Design review of the part built by this model. Coordinates are the model's own, in mm. Coordinates: 2 decimals unless noted, no trailing zeros. Write each loop counter-clockwise with the first axis right and the second up, starting at its lowest first coordinate (ties: lowest second). Pieces come first, ordered by that corner, then holes.
Q1. Add section A-A, the plane x = -35. Give the boundary of the cut face in (y, z), plus the area to 3 significant figures.
Q2. Add section C-C, the plane x = 365. Give the number of separate pieces and of enclosed holes in the cut face, plus the area to 3 significant figures.
Q3. To check wall thickness, follow probe 1 along X at (y, z) = (-37, 244); probe 2 along Z at (x, y) = (-161.5, -37); probe 3 along X at (y, z) = (-2, -305.5). State the ranges of each line that lie inside material, in increasing order.
Q4. Add section B-B, the plane z = -432. Give the boundary of the cut face in (x, y), plus the area to 3 significant figures.
from build123d import *

# Parameters (mm, degrees)
F0_W     = 1080
F0_H     = 2590
F0_W_2   = 20
F0_H_2   = 300
F0_W_3   = 340
F0_H_3   = 40
F0_H_4   = 420
F1_DEPTH = 40


# Not quite as in the source:
# - a feature names something its author has since deleted; it is built from what else it names


with BuildPart() as f1:
    # F0 (on Front) → F1 (new body)
    with BuildSketch(Plane.XZ):
        Rectangle(F0_W, F0_H)
        Polygon((520, -855), (520, -1275), (10, -1275), (-10, -1275), (-520, -1275), (-520, -855), (-520, -795), (-520, -495), (-520, -455), (-520, -155), (-520, -115), (-520, 595), (-520, 635), (-520, 935), (-520, 975), (-520, 1275), (160, 1275), (180, 1275), (520, 1275), (520, 975), (520, 935), (520, 635), (520, 595), (520, 339.328327179), (520, 299.328327179), (520, -115), (520, -155), (520, -455), (520, -495), (520, -795), align=None, mode=Mode.SUBTRACT)
        with Locations((170, 1125)):
            Rectangle(F0_W_2, F0_H_2)
        Polygon((-160, 935), (520, 935), (520, 975), (180, 975), (160, 975), (-520, 975), (-520, 935), (-180, 935), align=None)
        with Locations((-170, 785)):
            Rectangle(F0_W_2, F0_H_2)
        Polygon((180, 595), (520, 595), (520, 635), (-160, 635), (-180, 635), (-520, 635), (-520, 595), (160, 595), align=None)
        Polygon((160, -115), (180, -115), (180, 299.328327179), (180, 339.328327179), (180, 595), (160, 595), (160, 80), (160, 40), align=None)
        with Locations((350, 319.328327179)):
            Rectangle(F0_W_3, F0_H_3)
        Polygon((-160, -155), (520, -155), (520, -115), (180, -115), (160, -115), (-520, -115), (-520, -155), (-180, -155), align=None)
        with Locations((-170, -305)):
            Rectangle(F0_W_2, F0_H_2)
        Polygon((180, -495), (520, -495), (520, -455), (-160, -455), (-180, -455), (-520, -455), (-520, -495), (160, -495), align=None)
        with Locations((170, -645)):
            Rectangle(F0_W_2, F0_H_2)
        Polygon((10, -855), (520, -855), (520, -795), (180, -795), (160, -795), (-520, -795), (-520, -855), (-10, -855), align=None)
        with Locations((0, -1065)):
            Rectangle(F0_W_2, F0_H_4)
    extrude(amount=F1_DEPTH)


solid = f1.part
Here are the results:
1. outline: (-40, -1295) - (0, -1295) - (0, -1275) - (-40, -1275) - close; (-40, -855) - (0, -855) - (0, -795) - (-40, -795) - close; (-40, -495) - (0, -495) - (0, -455) - (-40, -455) - close; (-40, -155) - (0, -155) - (0, -115) - (-40, -115) - close; (-40, 595) - (0, 595) - (0, 635) - (-40, 635) - close; (-40, 935) - (0, 935) - (0, 975) - (-40, 975) - close; (-40, 1275) - (0, 1275) - (0, 1295) - (-40, 1295) - close
1. area: 10,400 mm2
2. separate pieces: 8
2. enclosed holes: 0
2. area: 12,000 mm2
3. probe 1: x = -540 to -520, 160 to 180, 520 to 540
3. probe 2: z = -1295 to -1275, -855 to -795, -495 to -115, 595 to 975, 1275 to 1295
3. probe 3: x = -540 to -520, -180 to -160, 520 to 540
4. outline: (-540, -40) - (-520, -40) - (-520, 0) - (-540, 0) - close; (-180, -40) - (-160, -40) - (-160, 0) - (-180, 0) - close; (520, -40) - (540, -40) - (540, 0) - (520, 0) - close
4. area: 2,400 mm2
